from build123d import *

# Parameters (mm, degrees)
SKETCH1_R                = 4
BOSS_EXTRUDE1_DEPTH      = 6
BOSS_EXTRUDE1_DEPTH_BACK = 6
SKETCH2_W                = 1.5
SKETCH2_H                = 5
CUT_EXTRUDE1_DEPTH       = 9


with BuildPart() as part:
    # Sketch1 → Boss-Extrude1 (new body, two sides)
    with BuildSketch(Plane(origin=(0, 0, 0), x_dir=(1, 0, 0), z_dir=(0, 1, 0))) as boss_extrude1_sk:
        with BuildLine():
            Line((-4, 3), (-7.5, 3))
            Line((-7.5, 3), (-7.5, -3))
            Line((-7.5, -3), (-4, -3))
            ThreePointArc((-4, -3), (5, 0), (-4, 3))
        make_face()
        Circle(SKETCH1_R, mode=Mode.SUBTRACT)
    extrude(amount=BOSS_EXTRUDE1_DEPTH)
    extrude(boss_extrude1_sk.sketch, amount=-BOSS_EXTRUDE1_DEPTH_BACK)

    # Sketch2 → Cut-Extrude1 (cut, through all)
    with BuildSketch(Plane(origin=(0, 0, -3), x_dir=(-1, 0, 0), z_dir=(0, 0, -1))):
        with Locations((5.15, 0)):
            Rectangle(SKETCH2_W, SKETCH2_H)
    extrude(amount=-CUT_EXTRUDE1_DEPTH, mode=Mode.SUBTRACT)


solid = part.part
Could you check a few things on this model? Use its own coordinates, in mm. A direction names the side the tool comes from. Give positions to 0.01 mm unless a question says otherwise; leave off trailing zeros. Order: outer loops, then holes, each group sorted by start corner. A loop starts at its lowest first (then second) coordinate and runs counter-clockwise, first axis right, second up. Notation, with made-up numbers: (38.25, 83.25) -> (68.25, 83.25) arc R27 cw to (68.25, 122.25) -> close; hole circle Ø5 at (3.25, 28). An arc over 180 degrees is marked (long way). Return JSON: item names as keys, results as strings.
1. Thinking about a two-plate mould opening in X: for faces 1 (the flat face through (-4.1, -6, 1)), 2 (the flat face through (-4.4, 0, 0)), 3 (the flat face through (-5, 2.5, 0)), 4 (the cylindrical face through (5, 0, 0)), which applies, pulls with the +X half, pulls with the -X half, needs draft (parallel to the pull), parting line crosses it, or undercut?
Answer list:
{"face 1": "needs draft", "face 2": "undercut", "face 3": "undercut", "face 4": "parting line crosses it"}
2. On a 3-axis mill with a long thin cutter (end or side, diameter ignored), from which of +Z, -Z, +X, -X, +Y, -Y can I reach the whole of each face in a straight line? I mean faces 5 (the flat face through (-4.1, 6, 1)), 6 (the flat face through (-5, -2.5, 0)), 7 (the flat face through (-6.2, 0.1, 3)), 8 (the flat face through (-6.1, 0.1, -3)). Say none if no direction works.
Answer list:
{"face 5": "+Z, -Z, +X, -X, +Y", "face 6": "+Z, -Z", "face 7": "+Z, -X, +Y, -Y", "face 8": "-Z, -X, +Y, -Y"}
3. Imagine slicing it at B-B on x = 0. List the corners of the cut face in (y, z) for me.
Answer list:
{"outline": "(-6, -5) -> (6, -5) -> (6, -4) -> (-6, -4) -> close; (-6, 4) -> (6, 4) -> (6, 5) -> (-6, 5) -> close"}
4. Imagine slicing it at D-D on y = -5.25. List the corners of the cut face in (x, z) for me.
Answer list:
{"outline": "(-7.5, -3) -> (-4, -3) arc R5 ccw (long way) to (-4, 3) -> (-7.5, 3) -> close; hole circle Ø8 at (0, 0)"}
5. I need wall thicknesses on line 1 (X direction, y = -1.7, z = 0); line 2 (Z direction, x = 0, y = -1.9); line 3 (X direction, y = 0.75, z = -2.75). Which ranges of each line are inside material? Lowest first, please. Write a range as from..to.
Answer list:
{"line 1": "x = -7.5..-5.9, -4.4..-4, 4..5", "line 2": "z = -5..-4, 4..5", "line 3": "x = -7.5..-5.9, -4.4..-2.9, 2.9..4.18"}
6. For pin 1 Ø1.8 at (x, y) = (-6, 2.5) entering from +Z; pin 2 Ø3 at (x, y) = (-5, -2.5) entering from -Z; pin 3 Ø3 at (y, z) = (-2.5, -2) entering from +X, each with a flat end and sliding along its axis, tell me the tip position at first contact or that it passes through.
Answer list:
{"pin 1": "stops at z = 3", "pin 2": "stops at z = -3.57", "pin 3": "stops at x = 4.97"}
7. Imagine slicing it at C-C on z = 0. List the corners of the cut face in (x, y) for me, then the cut area to 3 significant figures.
Answer list:
{"outline": "(-7.5, -6) -> (-4, -6) -> (-4, 6) -> (-7.5, 6) -> close; (4, -6) -> (5, -6) -> (5, 6) -> (4, 6) -> close; hole (-5.9, -2.5) -> (-4.4, -2.5) -> (-4.4, 2.5) -> (-5.9, 2.5) -> close", "area": "46.5 mm2"}
8. Imagine slicing it at A-A on y = -1.5. List the corners of the cut face in (x, z) for me.
Answer list:
{"outline": "(-7.5, -3) -> (-5.9, -3) -> (-5.9, 3) -> (-7.5, 3) -> close; (-4.4, -3) -> (-4, -3) arc R5 ccw (long way) to (-4, 3) -> (-4.4, 3) -> close; hole circle Ø8 at (0, 0)"}
